Design review of the part shown in the three views and the two pictorial views. Dimensions are in mm from the part's minimum x, y and z. A direction names the side the tool comes from. Coordinates: 2 decimals unless noted, no trailing zeros. Order: outer loops, then holes, each group sorted by start corner. A loop starts at its lowest first (then second) coordinate and runs counter-clockwise, first axis right, second up. Notation, with made-up numbers: (87, 30) - (129, 30) arc R22 ccw to (129, 59) - close; hole circle Ø7 at (49.5, -23.75). An arc over 180 degrees is marked (long way). One line per item, written item: value. Start each with the question number.
(1) For the marked faces 1 and 2, list the 3-axis set-ups (+Z, -Z, +X, -X, +Y, -Y) from which the entire face can be reached by the end or side of a thin tool; tool diameter is ignored.
(2) Consider section B-B on y = 60.5. Write out the cut boundary in (x, z), then the cut area to 3 significant figures.
(3) Consider section A-A on y = 25.5. Write out the cut boundary in (x, z), then the cut area to 3 significant figures.
(4) Clearance check with flat-ended pins moving along their axes: pin 1 (10 mm diameter, centred on x = 19, y = 18.5, fed in from -Z); pin 2 (8 mm diameter, centred on x = 23, z = 17.5, fed in from -Y); pin 3 (3 mm diameter, centred on y = 46.5, z = 24.5, fed in from +X). State where each tip first meets the part, or that it passes through.
(5) To check wall thickness, follow line 1 along Y through (x, z) = (6.75, 6); line 2 along Z through (x, y) = (25, 70.5); line 3 along Z through (x, y) = (4, 62). State the ranges of each line that lie inside material, in increasing order.
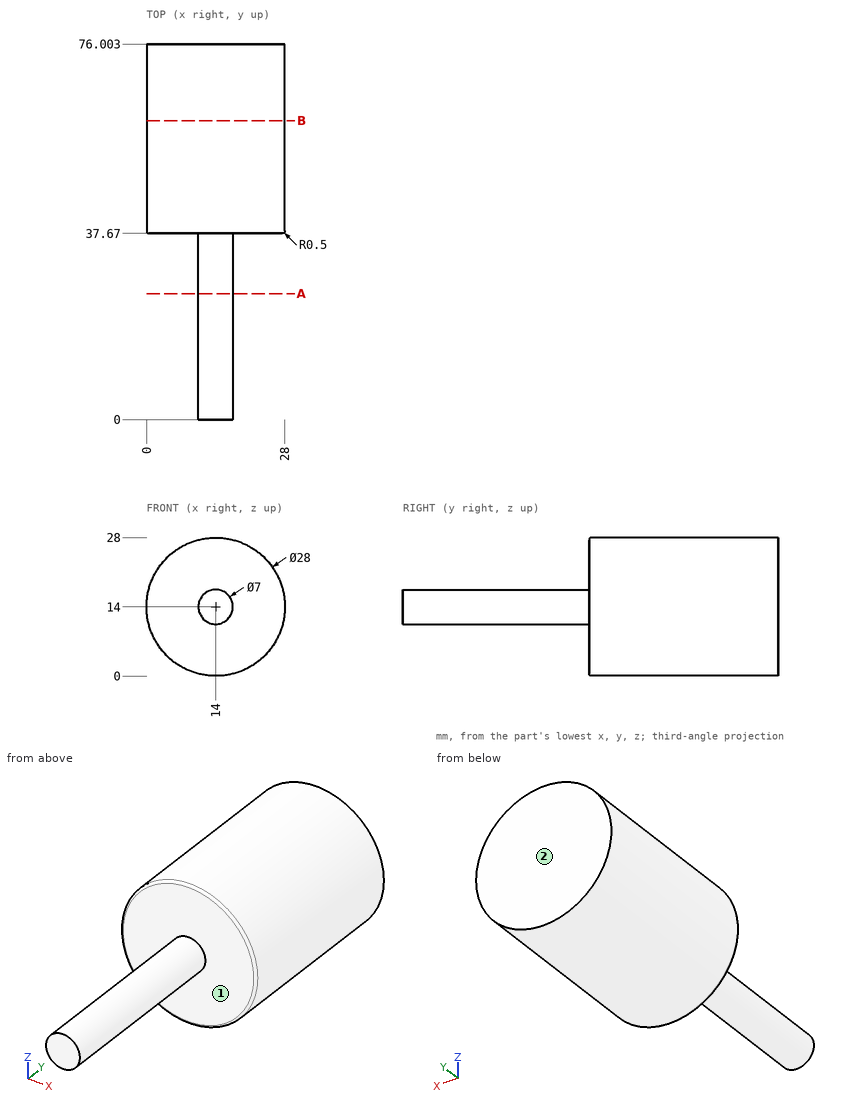
Geometry check:
1. face 1: -Y
1. face 2: +Z, -Z, +X, -X, +Y
2. outline: circle Ø28 at (14, 14)
2. area: 616 mm^2
3. outline: circle Ø7 at (14, 14)
3. area: 38.5 mm^2
4. pin 1: stops at z = 10.5
4. pin 2: stops at y = 37.67
4. pin 3: stops at x = 24.72
5. line 1: y = 37.67 to 76
5. line 2: z = 5.34 to 22.66
5. line 3: z = 4.2 to 23.8
